Part model, mm, in its own coordinate system. Face numbers are marked on the shaded views. A direction names the side the tool comes from. Round coordinates to 2 decimals unless told otherwise and drop trailing zeros. Order: outer loops, then holes, each group sorted by start corner. A loop starts at its lowest first (then second) coordinate and runs counter-clockwise, first axis right, second up. Notation, with made-up numbers: (44, 43.25) -> (57, 43.25) arc R17 ccw to (57, 70.25) -> close; hole circle Ø11 at (11.5, -25). An arc over 180 degrees is marked (long way). Answer as a JSON object with one key per item and string values. Group by question number.
```python
from build123d import *

# Parameters (mm, degrees)
F0_W      = 88.8
F0_H      = 26
F1_DEPTH  = 60
F3_DEPTH  = 45
F4_R      = 2
F5_W      = 88.9
F5_H      = 40
F6_DEPTH  = 10
F8_DEPTH  = 10
F9_R      = 2
F10_W     = 89
F10_H     = 45
F11_DEPTH = 15
F13_DEPTH = 5
F14_R     = 2
F15_R     = 4.6723110677
F15_R_2   = 4
F16_DEPTH = 85.001
F17_W     = 79.5239582658
F17_H     = 118.802215904
F18_DEPTH = 80
F19_R     = 3
F20_DEPTH = 3
F20_TAPER = 3
F21_DEPTH = 3
F21_TAPER = 3
F22_R     = 5.0890490665
F23_DEPTH = 25
F23_TAPER = -3


with BuildPart() as f1:
    # F0 (on Top) → F1 (new body)
    with BuildSketch(Plane.XY):
        Rectangle(F0_W, F0_H)
    extrude(amount=F1_DEPTH)

    # F2 (on face) → F3 (cut)
    with BuildSketch(Plane(origin=(0, 0, 0), x_dir=(1, 0, 0), z_dir=(0, 0, -1))):
        Polygon((-17.5, -7.6945363638), (0, -8), (17.5, -7.6945363638), (17.5, 7.6945363638), (0, 8), (-17.5, 7.6945363638), align=None)
    extrude(amount=-F3_DEPTH, mode=Mode.SUBTRACT)

    # F4
    f4_edges = [f1.edges().sort_by_distance(p)[0] for p in [
        (-17.5, 7.694536, 22.5),
        (-17.5, -7.694536, 22.5),
        (17.5, -7.694536, 22.5),
        (17.5, 7.694536, 22.5),
    ]]
    fillet(f4_edges, radius=F4_R)

    # F5 (on face) → F6 (join)
    with BuildSketch(Plane(origin=(0, 0, 0), x_dir=(1, 0, 0), z_dir=(0, 0, -1))):
        Rectangle(F5_W, F5_H)
    extrude(amount=F6_DEPTH)

    # F7 (on face) → F8 (cut)
    with BuildSketch(Plane(origin=(0, 0, -10), x_dir=(1, 0, 0), z_dir=(0, 0, -1))):
        Polygon((-20, -10.1508987014), (0, -10.5), (20, -10.1508987014), (20, 10.1508987014), (0, 10.5), (-20, 10.1508987014), align=None)
    extrude(amount=-F8_DEPTH, mode=Mode.SUBTRACT)

    # F9
    f9_edges = [f1.edges().sort_by_distance(p)[0] for p in [
        (-20, 10.150899, -5),
        (-20, -10.150899, -5),
        (20, 10.150899, -5),
        (20, -10.150899, -5),
    ]]
    fillet(f9_edges, radius=F9_R)

    # F10 (on face) → F11 (join)
    with BuildSketch(Plane(origin=(0, 0, -10), x_dir=(1, 0, 0), z_dir=(0, 0, -1))):
        Rectangle(F10_W, F10_H)
    extrude(amount=F11_DEPTH)

    # F12 (on face) → F13 (cut)
    with BuildSketch(Plane.XY.offset(-10)):
        Polygon((-39.5, -16.5605249353), (0, -17.25), (39.5, -16.5605249353), (39.5, 16.5605249353), (0, 17.25), (-39.5, 16.5605249353), align=None)
    extrude(amount=-F13_DEPTH, mode=Mode.SUBTRACT)

    # F14
    f14_edges = [f1.edges().sort_by_distance(p)[0] for p in [
        (-39.5, 16.560525, -12.5),
        (-39.5, -16.560525, -12.5),
        (39.5, -16.560525, -12.5),
        (39.5, 16.560525, -12.5),
    ]]
    fillet(f14_edges, radius=F14_R)

    # F15 (on face) → F16 (cut, through all)
    with BuildSketch(Plane.XY.offset(60)):
        with Locations((-27.5, 0)):
            Circle(F15_R)
        with Locations((27.5, 0)):
            Circle(F15_R_2)
    extrude(amount=-F16_DEPTH, mode=Mode.SUBTRACT)

    # F17 (on Right) → F18 (cut)
    with BuildSketch(Plane.YZ):
        with Locations((3.9665214717, 9.8679382354)):
            Rectangle(F17_W, F17_H)
    extrude(amount=-F18_DEPTH, mode=Mode.SUBTRACT)

    # F19 (on face) → F20 (join)
    with BuildSketch(Plane(origin=(0, 0, 0), x_dir=(0, -1, 0), z_dir=(-1, 0, 0))):
        with Locations((8.2831978798, 53.2280467451)):
            Circle(F19_R)
        with Locations((0, -20.896807313)):
            Circle(F19_R)
        with Locations((-8.2831978798, 53.2280467451)):
            Circle(F19_R)
    extrude(amount=F20_DEPTH, taper=F20_TAPER)

    # F19 (on face) → F21 (join)
    with BuildSketch(Plane(origin=(0, 0, 0), x_dir=(0, -1, 0), z_dir=(-1, 0, 0))):
        with Locations((8.2831978798, 53.2280467451)):
            Circle(F19_R)
        with Locations((0, -20.896807313)):
            Circle(F19_R)
        with Locations((-8.2831978798, 53.2280467451)):
            Circle(F19_R)
    extrude(amount=F21_DEPTH, taper=F21_TAPER)

    # F22 (on face) → F23 (cut)
    with BuildSketch(Plane(origin=(0, 0, 45), x_dir=(1, 0, 0), z_dir=(0, 0, -1))):
        Circle(F22_R)
    extrude(amount=-F23_DEPTH, taper=F23_TAPER, mode=Mode.SUBTRACT)


solid = f1.part
```
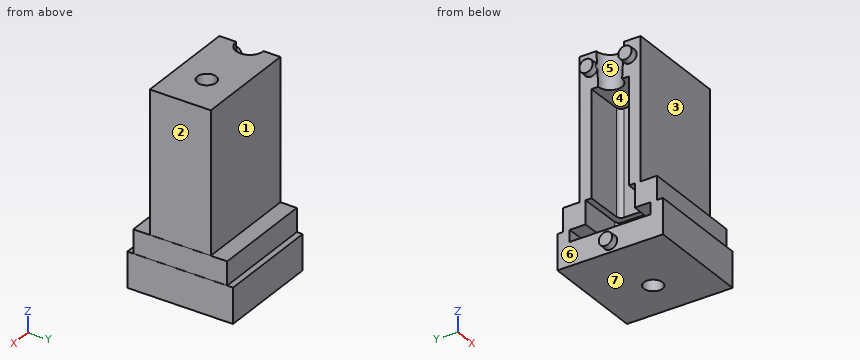
Q1. Drop flat-ended pins along their axis: pin 1 Ø5 at (x, z) = (11.5, -5) entering from -Y; pin 2 Ø12 at (y, z) = (4, 21) entering from +X; pin 3 Ø12 at (x, z) = (10, 19) entering from -Y. Give the stop position or say it passes through.
Q2. Which spindle directions (+Z, -Z, +X, -X, +Y, -Y) get a long thin tool onto all of the face, cutting with end or side? Do the marked faces 1, 2 and 3. Say none if no direction does.
Q3. Two-plate mould, pull along Z, no slides. Class the marked faces 4, 5, 6 and 7: +Z half, -Z half, draft (parallel to the pull), parting line (faces both ways), or undercut.
Q4. Band-saw the part on C-C (y = 0). List the corners of the cut face in (x, z), plus the area to 3 significant figures.
Q5. Band-saw the part on A-A (z = 29.5). List the corners of the cut face in (x, y).
Q6. Band-saw the part on D-D (x = 27.5). List the corners of the cut face in (y, z).
Q7. Band-saw the part on B-B (x = 34.5). List the corners of the cut face in (y, z).
Q8. Wall check: line 1 (Z direction, x = 29, y = -9); line 2 (Z direction, x = 4.5, y = 15.5); line 3 (Y direction, x = 27.5, z = -17.75). Give the ranges that are in metal, low to high. Write a range as [from, to].
Completed:
{
 "1": {"pin 1": "y = -20", "pin 2": "x = 44.4", "pin 3": "y = -13"},
 "2": {"face 1": "+Z, +X, -X, +Y", "face 2": "+Z, +X, +Y, -Y", "face 3": "+Z, +X, -X, -Y"},
 "3": {"face 4": "undercut", "face 5": "+Z half", "face 6": "draft", "face 7": "-Z half"},
 "4": {"outline": "(-3, -23.74) -> (0, -23.9) -> (0, -25) -> (23.5, -25) -> (23.5, -15) -> (0, -15) -> (0, -17.9) -> (-3, -18.05) -> close; (5.09, 45) -> (17.5, 45) -> (17.5, 0) -> (20, 0) -> (20, -10) -> (23.5, -10) -> (23.5, 60) -> (5.88, 60) -> close; (31.5, -25) -> (44.5, -25) -> (44.5, -10) -> (44.45, -10) -> (44.45, 0) -> (44.4, 0) -> (44.4, 60) -> (31.5, 60) -> (31.5, -10) -> (39.5, -10) -> (39.5, -15) -> (31.5, -15) -> close", "area": "1,890 mm2"},
 "5": {"outline": "(0, -13) -> (44.4, -13) -> (44.4, 13) -> (0, 13) -> (0, 8) -> (15.53, 7.73) arc R2 cw to (17.5, 5.73) -> (17.5, -5.73) arc R2 cw to (15.53, -7.73) -> (0, -8) -> close; hole circle Ø8 at (27.5, 0)"},
 "6": {"outline": "(-22.5, -25) -> (-4, -25) -> (-4, -15) -> (-16.77, -15) -> (-16.77, -10) -> (-4, -10) -> (-4, 60) -> (-13, 60) -> (-13, 0) -> (-20, 0) -> (-20, -10) -> (-22.5, -10) -> close; (4, -25) -> (22.5, -25) -> (22.5, -10) -> (20, -10) -> (20, 0) -> (13, 0) -> (13, 60) -> (4, 60) -> (4, -10) -> (16.77, -10) -> (16.77, -15) -> (4, -15) -> close"},
 "7": {"outline": "(-22.5, -25) -> (22.5, -25) -> (22.5, -10) -> (20, -10) -> (20, 0) -> (13, 0) -> (13, 60) -> (-13, 60) -> (-13, 0) -> (-20, 0) -> (-20, -10) -> (-22.5, -10) -> close; hole (-16.65, -15) -> (16.65, -15) -> (16.65, -10) -> (-16.65, -10) -> close"},
 "8": {"line 1": "[-25, -15], [-10, 60]", "line 2": "[-25, -15], [-10, 0]", "line 3": "[-22.5, -4], [4, 22.5]"}
}
